```python
from build123d import *
from build123d.topology import SkipClean

# Parameters (mm, degrees)
SKETCH1_R           = 16
BOSS_EXTRUDE1_DEPTH = 17
FILLET1_R           = 1.5
BOSS_EXTRUDE2_START = 3
BOSS_EXTRUDE2_DEPTH = 3
CIRPATTERN1_COUNT   = 4
FILLET2_R           = 1.5
SKETCH5_R           = 3
BOSS_EXTRUDE3_DEPTH = 3
FILLET3_R           = 0.5
SKETCH6_R           = 19
BOSS_EXTRUDE4_DEPTH = 20.5
CHAMFER1_SIZE       = 1
SKETCH7_W           = 4
SKETCH7_H           = 0.5
BOSS_EXTRUDE5_DEPTH = 4
FILLET4_R           = 2
FILLET5_R           = 2
SKETCH8_R           = 6.6
BOSS_EXTRUDE6_DEPTH = 12
BOSS_EXTRUDE7_START = 21.5
SKETCH9_R           = 3
BOSS_EXTRUDE7_DEPTH = 21.5
CHAMFER2_SIZE       = 0.6
CHAMFER3_SIZE       = 0.6


with BuildPart() as part:
    # Sketch1 → Boss-Extrude1 (new body)
    with BuildSketch(Plane.XY):
        Circle(SKETCH1_R)
    extrude(amount=BOSS_EXTRUDE1_DEPTH)

    # Fillet1
    fillet1_edges = [part.edges().sort_by_distance(p)[0] for p in [
        (-16, 0, 17),
    ]]
    fillet(fillet1_edges, radius=FILLET1_R)

    # Sketch3 → Boss-Extrude2 (add)
    with SkipClean():  # the faces are left unmerged after this step: merging them gives an invalid solid
        with BuildSketch(Plane(origin=(0, 0, 0), x_dir=(-1, 0, 0), z_dir=(0, 0, -1)).offset(BOSS_EXTRUDE2_START)):
            with BuildLine():
                Line((-2.5, 15.803481), (-2.5, -15.803481))
                ThreePointArc((-2.5, -15.803481), (0, -16), (2.5, -15.803481))
                Line((2.5, -15.803481), (2.5, 15.803481))
                ThreePointArc((2.5, 15.803481), (0, 16), (-2.5, 15.803481))
            make_face()
        boss_extrude2 = extrude(amount=-BOSS_EXTRUDE2_DEPTH)

    # CirPattern1: Boss-Extrude2 ×4 about axis
    with SkipClean():  # the faces are left unmerged after this step: merging them gives an invalid solid
        cirpattern1_axis = Axis((0, 0, 0), (0, 0, -1))
        for i in range(1, CIRPATTERN1_COUNT):
            add(boss_extrude2.rotate(cirpattern1_axis, i * 360 / CIRPATTERN1_COUNT))

    # Fillet2
    fillet2_edges = [part.edges().sort_by_distance(p)[0] for p in [
        (-2.5, 2.5, -1.5),
        (2.5, 2.5, -1.5),
        (-2.5, -2.5, -1.5),
        (2.5, -2.5, -1.5),
    ]]
    fillet(fillet2_edges, radius=FILLET2_R)

    # Sketch5 → Boss-Extrude3 (add)
    with SkipClean():  # the faces are left unmerged after this step: merging them gives an invalid solid
        with BuildSketch(Plane(origin=(0, 0, -3), x_dir=(-1, 0, 0), z_dir=(0, 0, -1))):
            Circle(SKETCH5_R)
        extrude(amount=BOSS_EXTRUDE3_DEPTH)

    # Fillet3
    fillet3_edges = [part.edges().sort_by_distance(p)[0] for p in [
        (3, 0, -6),
    ]]
    fillet(fillet3_edges, radius=FILLET3_R)

    # Sketch6 → Boss-Extrude4 (add)
    with SkipClean():  # the faces are left unmerged after this step: merging them gives an invalid solid
        with BuildSketch(Plane.XY.offset(17)):
            Circle(SKETCH6_R)
        extrude(amount=BOSS_EXTRUDE4_DEPTH)

    # Chamfer1
    chamfer1_edges = [part.edges().sort_by_distance(p)[0] for p in [
        (-19, 0, 17),
    ]]
    chamfer(chamfer1_edges, length=CHAMFER1_SIZE)

    # Sketch7 → Boss-Extrude5 (add)
    with SkipClean():  # the faces are left unmerged after this step: merging them gives an invalid solid
        with BuildSketch(Plane(origin=(0, 0, -3), x_dir=(-1, 0, 0), z_dir=(0, 0, -1))):
            with Locations((12, 0)):
                Rectangle(SKETCH7_W, SKETCH7_H)
            with Locations((-12, 0)):
                Rectangle(SKETCH7_W, SKETCH7_H)
        extrude(amount=BOSS_EXTRUDE5_DEPTH)

    # Fillet4
    fillet4_edges = [part.edges().sort_by_distance(p)[0] for p in [
        (14, 0, -7),
        (10, 0, -7),
        (-10, 0, -7),
        (-14, 0, -7),
    ]]
    fillet(fillet4_edges, radius=FILLET4_R - 0.0001)  # a hair under: the kernel refuses the full size

    # Fillet5
    fillet5_edges = [part.edges().sort_by_distance(p)[0] for p in [
        (-19, 0, 37.5),
    ]]
    fillet(fillet5_edges, radius=FILLET5_R)

    # Sketch8 → Boss-Extrude6 (add)
    with BuildSketch(Plane.XY.offset(37.5)):
        Circle(SKETCH8_R)
    extrude(amount=BOSS_EXTRUDE6_DEPTH)

    # Sketch9 → Boss-Extrude7 (add)
    with BuildSketch(Plane.XY.offset(49.5).offset(BOSS_EXTRUDE7_START)):
        with Locations(Location((0, 0, 0), (0, 0, 180))):
            Circle(SKETCH9_R)
    extrude(amount=-BOSS_EXTRUDE7_DEPTH)

    # Chamfer2
    chamfer2_edges = [part.edges().sort_by_distance(p)[0] for p in [
        (3, 0, 71),
    ]]
    chamfer(chamfer2_edges, length=CHAMFER2_SIZE)

    # Chamfer3
    chamfer3_edges = [part.edges().sort_by_distance(p)[0] for p in [
        (-6.6, 0, 49.5),
    ]]
    chamfer(chamfer3_edges, length=CHAMFER3_SIZE)


solid = part.part
```
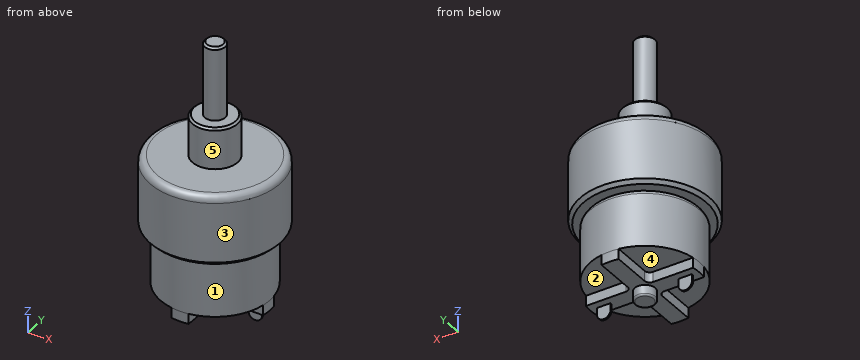
The listing builds one solid part. Answer for the finished solid, in the listing's coordinates (mm). Face numbers are marked on the shaded views. A direction names the side the tool comes from. Round coordinates to 2 decimals unless told otherwise and drop trailing zeros. Loops run counter-clockwise (first coordinate to the right, second up) from the corner with the lowest first, then second, coordinate; pieces in that order, holes last. Notation, with made-up numbers: (28, 14.5) - (87, 14.5) arc R10 cw to (87, 18.5) - close; hole circle Ø8 at (-35, -20). An arc over 180 degrees is marked (long way). Return JSON: item names as keys, results as strings. Group by question number.
1. Each of these flat-tipped pins is pushed along its axis until it touches: P1, Ø1.5, axis at x = -10, z = -1, coming from the -Y side; P2, Ø1.5, axis at y = 9.5, z = -2, coming from the +X side; P3, Ø14.5, axis at x = -11, y = 10, coming from the -Z side. Where does it stop, or does it pass through?
2. Which of the six approach directions +Z, -Z, +X, -X, +Y, -Y give full straight-line access (tool end or side, diameter ignored) to the marked faces 1, 2, 3, 4 and 5?
3. The part is cut by section C-C on z = 57. Determine the outline of the cut face in (x, y).
4. The part is cut by section B-B on z = 26.5. Determine the outline of the cut face in (x, y).
5. Consider probe 1 along Z at (x, y) = (-1.5, 12); probe 2 along Z at (x, y) = (9, 7.5); probe 3 along Z at (x, y) = (-9, -13). Determine where each line is inside the solid, lowest interval first.
Resolved:
{
 "1": {"P1": "stops at y = -2.5", "P2": "stops at x = 2.5", "P3": "stops at z = 0"},
 "2": {"face 1": "-Z", "face 2": "-Z, +X, +Y", "face 3": "+Z, -Z", "face 4": "-Z, -X, +Y", "face 5": "+Z"},
 "3": {"outline": "circle Ø6 at (0, 0)"},
 "4": {"outline": "circle Ø38 at (0, 0)"},
 "5": {"probe 1": "z = -3 to 37.5", "probe 2": "z = 0 to 37.5", "probe 3": "z = 0 to 16.23, 17 to 37.5"}
}
